Here's how the part is built. I have some questions about the finished solid (model axes, mm). Face numbers are marked on the shaded views. A direction names the side the tool comes from. Round coordinates to 2 decimals unless told otherwise and drop trailing zeros. Write each loop counter-clockwise with the first axis right and the second up, starting at its lowest first coordinate (ties: lowest second). Pieces come first, ordered by that corner, then holes. Notation, with made-up numbers: (20.5, 48.5) - (58.5, 48.5) arc R25 ccw to (58.5, 64.5) - close; hole circle Ø3 at (30.25, 43.25). An arc over 180 degrees is marked (long way). Use one line per item in the form item = value. Start each with the question number.
1. I want a section at A-A, the plane y = 0. List the corners of the cut face in (x, z) for me, plus the area to 3 significant figures.
2. Will these pins go through, and if not, where does the flat tip stop? pin 1 (12 mm diameter, centred on x = -2.5, y = 2.5, fed in from +Z); pin 2 (4 mm diameter, centred on y = -2.5, z = 5.5, fed in from -X); pin 3 (3 mm diameter, centred on y = 3, z = 9.5, fed in from -X).
3. I want a section at C-C, the plane z = 5.5. List the corners of the cut face in (x, y) for me.
4. I want a section at D-D, the plane z = 3. List the corners of the cut face in (x, y) for me.
5. If I drill on line 1 along Y through (x, z) = (0, 5); line 2 along Y through (x, z) = (0, 7); line 3 along X through (y, z) = (-0.5, 7), over which ranges is the centre line in solid material (lowest first)?
6. We'd pull the mould along X, two halves only. Please class the marked faces 3, 4 and 5: +X half, -X half, draft (parallel to the pull), parting line (faces both ways), or undercut.
7. Which directions (+Z, -Z, +X, -X, +Y, -Y) give clear straight access to the entire face, cutting with the end or side of a thin tool? Please do the marked faces 1 and 2.
```python
from build123d import *

# Parameters (mm, degrees)
F0_R     = 8.55
F1_DEPTH = 11
F0_R_2   = 12
F2_DEPTH = 6
F3_R     = 5.1
F4_DEPTH = 25
F5_SIZE  = 0.8


with BuildPart() as f1:
    # F0 (on Top) → F1 (new body)
    with BuildSketch(Plane.XY):
        Circle(F0_R)
    extrude(amount=F1_DEPTH)

    # F0 (on Top) → F2 (join)
    with BuildSketch(Plane.XY):
        Circle(F0_R_2)
        Circle(F0_R, mode=Mode.SUBTRACT)
    extrude(amount=F2_DEPTH)

    # F3 (on face) → F4 (cut)
    with BuildSketch(Plane.XY.offset(11)):
        Circle(F3_R)
    extrude(amount=-F4_DEPTH, mode=Mode.SUBTRACT)

    # F5
    f5_edges = [f1.edges().sort_by_distance(p)[0] for p in [
        (-12, 0, 6),
    ]]
    chamfer(f5_edges, length=F5_SIZE)


solid = f1.part
```
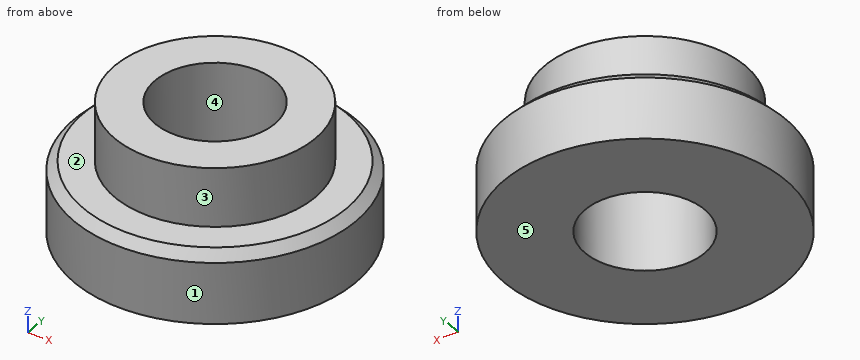
Model answer:
q1.outline = (-12, 0) - (-5.1, 0) - (-5.1, 11) - (-8.55, 11) - (-8.55, 6) - (-11.2, 6) - (-12, 5.2) - close; (5.1, 0) - (12, 0) - (12, 5.2) - (11.2, 6) - (8.55, 6) - (8.55, 11) - (5.1, 11) - close
q1.area = 117 mm2
q2.pin_1 = 11
q2.pin_2 = -11.99
q2.pin_3 = -8.42
q3.outline = circle Ø23.4 at (0, 0); hole circle Ø10.2 at (0, 0)
q4.outline = circle Ø24 at (0, 0); hole circle Ø10.2 at (0, 0)
q5.line_1 = -12 to -5.1, 5.1 to 12
q5.line_2 = -8.55 to -5.1, 5.1 to 8.55
q5.line_3 = -8.54 to -5.08, 5.08 to 8.54
q6.face_3 = parting line
q6.face_4 = undercut
q6.face_5 = draft
q7.face_1 = +Z, -Z
q7.face_2 = +Z
